The listing builds one solid part. Answer for the finished solid, in the listing's coordinates (mm). A direction names the side the tool comes from. Give positions to 0.01 mm unless a question says otherwise; leave off trailing zeros. Loops run counter-clockwise (first coordinate to the right, second up) from the corner with the lowest first, then second, coordinate; pieces in that order, holes last. Notation, with made-up numbers: (-25, 55.5) -> (-20, 55.5) arc R19 cw to (-20, 86.5) -> close; hole circle Ø11 at (-39.5, 46). An arc over 180 degrees is marked (long way). One line per question, with ' | ' between items. Start each with the question number.
from build123d import *

# Parameters (mm, degrees)
BOSS_EXTRUDE1_DEPTH = 1.2
FILLET1_R           = 5
FILLET2_R           = 0.8


with BuildPart() as part:
    # Sketch1 → Boss-Extrude1 (new body)
    with BuildSketch(Plane.XY):
        with BuildLine():
            Line((-10.5, 0), (-12.5, -2))
            Line((-12.5, -2), (-12, -12))
            Line((-12, -12), (-12.5, -14))
            Line((-12.5, -14), (-14.5, -14))
            Line((-14.5, -14), (-14.5, 3))
            Line((-14.5, 3), (-12.5, 3))
            Line((-12.5, 3), (12.5, 3))
            Line((12.5, 3), (14.5, 3))
            Line((14.5, 3), (14.5, -14))
            Line((14.5, -14), (12.5, -14))
            Line((12.5, -14), (12, -12))
            Line((12, -12), (12.5, -2))
            Line((12.5, -2), (10.5, 0))
            Line((10.5, 0), (8, 0))
            Line((8, 0), (8, -12))
            Line((8, -12), (3.5, -12))
            Line((3.5, -12), (3.5, -7))
            ThreePointArc((3.5, -7), (0, -3.5), (-3.5, -7))
            Line((-3.5, -7), (-3.5, -12))
            Line((-3.5, -12), (-8, -12))
            Line((-8, -12), (-8, 0))
            Line((-8, 0), (-10.5, 0))
        make_face()
    extrude(amount=BOSS_EXTRUDE1_DEPTH)

    # Fillet1
    fillet1_edges = [part.edges().sort_by_distance(p)[0] for p in [
        (-12, -12, 0.6),
        (12, -12, 0.6),
    ]]
    fillet(fillet1_edges, radius=FILLET1_R)

    # Fillet2
    fillet2_edges = [part.edges().sort_by_distance(p)[0] for p in [
        (-12.5, -14, 0.6),
        (-14.5, -14, 0.6),
        (-14.5, 3, 0.6),
        (14.5, 3, 0.6),
        (14.5, -14, 0.6),
        (12.5, -14, 0.6),
        (8, -12, 0.6),
        (3.5, -12, 0.6),
        (-3.5, -12, 0.6),
        (-8, -12, 0.6),
    ]]
    fillet(fillet2_edges, radius=FILLET2_R)


solid = part.part
1. Determine the mould class of faces 1 (the cylindrical face through (-14.27, 2.76, 0.61)), 2 (the flat face through (-9, 0, 1)), 3 (the flat face through (-12.27, -6.56, 0.59)) for opening direction Y: released by +Y, released by -Y, zero draft, split by the parting line, or undercut.
2. Straight lines are drawn through the part: L1, parallel to X at y = -5.5, z = 0.3 (3 decimals); L2, parallel to X at y = -4.75, z = 0.2; L3, parallel to Y at x = 7, z = 0.2. For each, find the intervals that lie inside material, in ascending order.
3. The part is cut by section C-C (x = -11.75). Write down the section's boundary in (y, z).
4. The part is cut by section B-B (x = 4.75). Write down the section's boundary in (y, z).
5. Each of these flat-tipped pins is pushed along its axis until it touches: pin 1 Ø0.6 at (x, z) = (9.5, 0.5) entering from -Y; pin 2 Ø1 at (x, y) = (-11.5, -11.5) entering from +Z. Where does it stop, or does it pass through?
6. The part is cut by section A-A (y = -2.5). Write down the section's boundary in (x, z) (3 decimals).
7. For faces 4 (the flat face through (11.5, -1, 0.6)), 5 (the flat face through (-14.5, -6, 1)), 6 (the cylindrical face through (-3.74, -11.77, 0.61)), determine the directions among +Z, -Z, +X, -X, +Y, -Y from which every point of the face is accessible in a straight line to the end or side of a thin tool.
Check sheet entries:
1) face 1: released by +Y | face 2: released by -Y | face 3: undercut
2) L1: x = -14.5 to -12.325, -8 to -3.162, 3.162 to 8, 12.325 to 14.5 | L2: x = -14.5 to -12.36, -8 to -2.68, 2.68 to 8, 12.36 to 14.5 | L3: y = -12 to 3
3) outline: (-1.25, 0) -> (3, 0) -> (3, 1.2) -> (-1.25, 1.2) -> close
4) outline: (-12, 0) -> (3, 0) -> (3, 1.2) -> (-12, 1.2) -> close
5) pin 1: stops at y = 0 | pin 2: passes through
6) outline: (-14.5, 0) -> (-12.475, 0) -> (-12.475, 1.2) -> (-14.5, 1.2) -> close; (-8, 0) -> (8, 0) -> (8, 1.2) -> (-8, 1.2) -> close; (12.475, 0) -> (14.5, 0) -> (14.5, 1.2) -> (12.475, 1.2) -> close
7) face 4: +Z, -Z | face 5: +Z, -Z, -X, +Y, -Y | face 6: +Z, -Z, -Y
